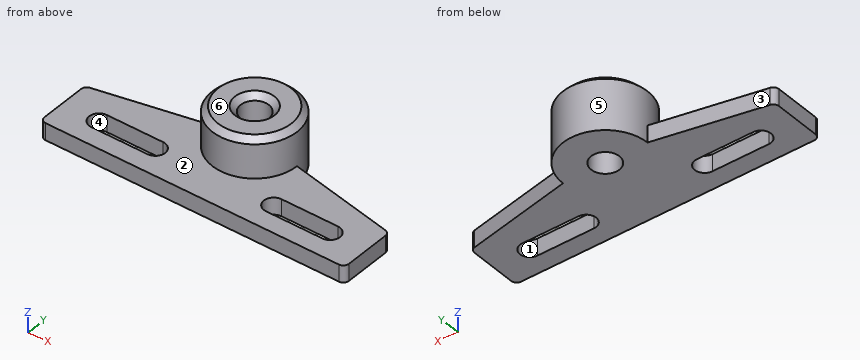
```python
from build123d import *

# Parameters (mm, degrees)
SKETCH_R        = 2.5
PAD_DEPTH       = 3
SKETCH001_R     = 7.5
SKETCH001_R_2   = 2.5
PAD001_DEPTH    = 7
CHAMFER_SIZE    = 1
FILLET_R        = 1
FILLET001_R     = 1
FILLET002_R     = 1
FILLET003_R     = 1
CHAMFER001_SIZE = 1


with BuildPart() as part:
    # Sketch → Pad (new body)
    with BuildSketch(Plane.XY):
        with BuildLine():
            Line((-27, -5), (27, -5))
            Line((27, -5), (27, 5))
            Line((7.5, 9), (27, 5))
            ThreePointArc((7.5, 9), (0, 16.5), (-7.5, 9))
            Line((-27, 5), (-7.5, 9))
            Line((-27, 5), (-27, -5))
        make_face()
        with Locations((0, 9)):
            Circle(SKETCH_R, mode=Mode.SUBTRACT)
        with BuildLine():
            ThreePointArc((-20.5, 1.75), (-22.25, 0), (-20.5, -1.75))
            Line((-20.5, -1.75), (-10.5, -1.75))
            ThreePointArc((-10.5, -1.75), (-8.75, 0), (-10.5, 1.75))
            Line((-20.5, 1.75), (-10.5, 1.75))
        make_face(mode=Mode.SUBTRACT)
        with BuildLine():
            ThreePointArc((20.5, -1.75), (22.25, 0), (20.5, 1.75))
            Line((20.5, 1.75), (10.5, 1.75))
            ThreePointArc((10.5, 1.75), (8.75, 0), (10.5, -1.75))
            Line((20.5, -1.75), (10.5, -1.75))
        make_face(mode=Mode.SUBTRACT)
    extrude(amount=PAD_DEPTH)

    # Sketch001 (on Face17 of Pad) → Pad001 (join)
    with BuildSketch(Plane.XY.offset(3)):
        with Locations((0, 9)):
            Circle(SKETCH001_R)
        with Locations((0, 9)):
            Circle(SKETCH001_R_2, mode=Mode.SUBTRACT)
    extrude(amount=PAD001_DEPTH)

    # Chamfer
    chamfer_edges = [part.edges().sort_by_distance(p)[0] for p in [
        (-2.5, 9, 10),
    ]]
    chamfer(chamfer_edges, length=CHAMFER_SIZE)

    # Fillet
    fillet_edges = [part.edges().sort_by_distance(p)[0] for p in [
        (27, -5, 1.5),
    ]]
    fillet(fillet_edges, radius=FILLET_R)

    # Fillet001
    fillet001_edges = [part.edges().sort_by_distance(p)[0] for p in [
        (-27, -5, 1.5),
    ]]
    fillet(fillet001_edges, radius=FILLET001_R)

    # Fillet002
    fillet002_edges = [part.edges().sort_by_distance(p)[0] for p in [
        (27, 5, 1.5),
    ]]
    fillet(fillet002_edges, radius=FILLET002_R)

    # Fillet003
    fillet003_edges = [part.edges().sort_by_distance(p)[0] for p in [
        (-27, 5, 1.5),
    ]]
    fillet(fillet003_edges, radius=FILLET003_R)

    # Chamfer001
    chamfer001_edges = [part.edges().sort_by_distance(p)[0] for p in [
        (-7.5, 9, 10),
    ]]
    chamfer(chamfer001_edges, length=CHAMFER001_SIZE)


solid = part.part
```
The listing builds one solid part. Answer for the finished solid, in the listing's coordinates (mm). Face numbers are marked on the shaded views. A direction names the side the tool comes from. Round coordinates to 2 decimals unless told otherwise and drop trailing zeros. Loops run counter-clockwise (first coordinate to the right, second up) from the corner with the lowest first, then second, coordinate; pieces in that order, holes last. Notation, with made-up numbers: (6.25, -35) -> (18.25, -35) arc R33 cw to (18.25, 0) -> close; hole circle Ø4 at (35, 20.25). An arc over 180 degrees is marked (long way). Use one line per item in the form item = value.
1. Flat-ended cylindrical pins translate along their axes: pin 1 Ø8 at (x, y) = (0, 9) entering from -Z; pin 2 Ø5 at (x, z) = (14.5, 2) entering from +Y; pin 3 Ø6 at (x, y) = (-5, -0.5) entering from +Z; pin 4 Ø0.9 at (x, z) = (17.5, 1.5) entering from +Y. Find the tip coordinate at first contact, or state that the pin passes through.
Answer key:
pin_1 = 0
pin_2 = 8.08
pin_3 = 3
pin_4 = 7.04
2. The part is cut by section C-C on y = 0. Determine the outline of the cut face in (x, z).
Answer key:
outline = (-27, 0) -> (-22.25, 0) -> (-22.25, 3) -> (-27, 3) -> close; (-8.75, 0) -> (8.75, 0) -> (8.75, 3) -> (-8.75, 3) -> close; (22.25, 0) -> (27, 0) -> (27, 3) -> (22.25, 3) -> close
3. A tool of negligible diameter and unlimited length cuts with its end or side. For the marked faces 5 and 6, from which of +Z, -Z, +X, -X, +Y, -Y can it reach the whole face along a straight path? Write none if from no direction.
Answer key:
face_5 = +Z
face_6 = +Z, +X, -X, +Y, -Y
4. Find the intervals of material crossed by probe 1 along Y at (x, z) = (0, 6); probe 2 along Z at (x, y) = (-6, -2.25); probe 3 along Y at (x, z) = (-17, 0.75), in increasing order. Write a range as [from, to].
Answer key:
probe_1 = [1.5, 6.5], [11.5, 16.5]
probe_2 = [0, 3]
probe_3 = [-5, -1.75], [1.75, 7.05]
5. The part is cut by section A-A on x = 0. Determine the outline of the cut face in (y, z).
Answer key:
outline = (-5, 0) -> (6.5, 0) -> (6.5, 9) -> (5.5, 10) -> (2.5, 10) -> (1.5, 9) -> (1.5, 3) -> (-5, 3) -> close; (11.5, 0) -> (16.5, 0) -> (16.5, 9) -> (15.5, 10) -> (12.5, 10) -> (11.5, 9) -> close
6. The part is cut by section D-D on x = 17. Determine the outline of the cut face in (y, z).
Answer key:
outline = (-5, 0) -> (-1.75, 0) -> (-1.75, 3) -> (-5, 3) -> close; (1.75, 0) -> (7.05, 0) -> (7.05, 3) -> (1.75, 3) -> close
7. For a pull along Y with two mould halves and no side action, classify the marked faces 1, 2, 3 and 4 as released by +Y, released by -Y, zero draft, split by the parting line, or undercut.
Answer key:
face_1 = undercut
face_2 = zero draft
face_3 = released by +Y
face_4 = undercut
8. The part is cut by section B-B on z = 1. Determine the outline of the cut face in (x, y).
Answer key:
outline = (-27, -4) arc R1 ccw to (-26, -5) -> (26, -5) arc R1 ccw to (27, -4) -> (27, 4.18) arc R1 ccw to (26.2, 5.16) -> (7.5, 9) arc R7.5 ccw to (-7.5, 9) -> (-26.2, 5.16) arc R1 ccw to (-27, 4.18) -> close; hole (-20.5, -1.75) -> (-10.5, -1.75) arc R1.75 ccw to (-10.5, 1.75) -> (-20.5, 1.75) arc R1.75 ccw to start; hole circle Ø5 at (0, 9); hole (10.5, -1.75) -> (20.5, -1.75) arc R1.75 ccw to (20.5, 1.75) -> (10.5, 1.75) arc R1.75 ccw to start
